Check sheet for the modelled part. Datum: model origin and axes. Units: mm. Face numbers are marked on the shaded views. A direction names the side the tool comes from. Give positions to 0.01 mm unless a question says otherwise; leave off trailing zeros. Order: outer loops, then holes, each group sorted by start corner. A loop starts at its lowest first (then second) coordinate and runs counter-clockwise, first axis right, second up. Notation, with made-up numbers: M 12.25,23 L 65.25,23 A9 cw 65.25,38 Z; hole C 82.25,5 d4. An arc over 180 degrees is marked long. Return JSON: item names as keys, results as strings. Group by question number.
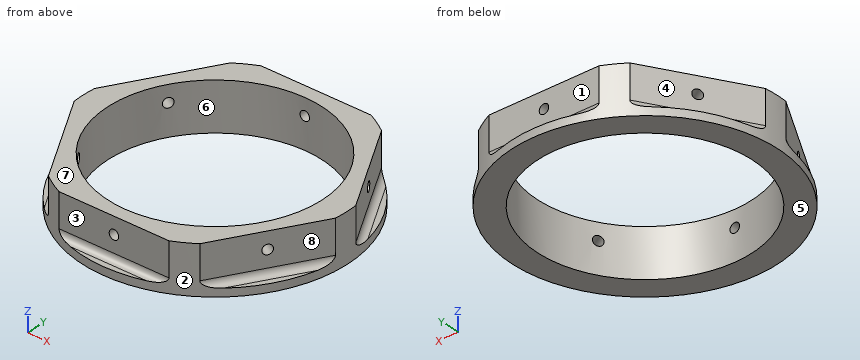
from build123d import *

# Parameters (mm, degrees)
SZKIC2_R                    = 46.017617149
DODANIE_WYCI_GNI_CIE1_DEPTH = 2.5
DODANIE_WYCI_GNI_CIE2_DEPTH = 15
SZKIC3_R                    = 46.5
SZKIC3_R_2                  = 42.5
WYTNIJ_WYCI_GNI_CIE3_DEPTH  = 10
SZKIC8_R                    = 33.35
WYTNIJ_WYCI_GNI_CIE2_DEPTH  = 62.947558467
ZAOKR_GLENIE2_R             = 2
SZKIC9_R                    = 1.5
WYTNIJ_WYCI_GNI_CIE4_DEPTH  = 10
SZYK_KO_OWY1_COUNT          = 6
SZKIC10_R                   = 50
SZKIC10_R_2                 = 41.3
WYTNIJ_WYCI_GNI_CIE5_DEPTH  = 62.947558491


with BuildPart() as part:
    # Szkic2 → Dodanie-wyci_gni_cie1 (new body)
    with BuildSketch(Plane.XY):
        Circle(SZKIC2_R)
    extrude(amount=DODANIE_WYCI_GNI_CIE1_DEPTH)

    # Szkic2_3 → Dodanie-wyci_gni_cie2 (add)
    with BuildSketch(Plane.XY):
        with BuildLine():
            ThreePointArc((17.776388835, -37.5), (20.75, -35.940054257), (23.587758225, -34.144804318))
            Line((23.587758225, -34.144804318), (41.364147059, -3.355195682))
            ThreePointArc((41.364147059, -3.355195682), (41.466022856, -1.67897246), (41.5, 0))
            ThreePointArc((41.5, 0), (41.466022856, 1.67897246), (41.364147059, 3.355195682))
            Line((41.364147059, 3.355195682), (23.587758225, 34.144804318))
            ThreePointArc((23.587758225, 34.144804318), (20.75, 35.940054257), (17.776388835, 37.5))
            Line((17.776388835, 37.5), (-17.776388835, 37.5))
            ThreePointArc((-17.776388835, 37.5), (-20.75, 35.940054257), (-23.587758225, 34.144804318))
            Line((-23.587758225, 34.144804318), (-41.364147059, 3.355195682))
            ThreePointArc((-41.364147059, 3.355195682), (-41.5, 0), (-41.364147059, -3.355195682))
            Line((-41.364147059, -3.355195682), (-23.587758225, -34.144804318))
            ThreePointArc((-23.587758225, -34.144804318), (-20.75, -35.940054257), (-17.776388835, -37.5))
            Line((-17.776388835, -37.5), (17.776388835, -37.5))
        make_face()
    extrude(amount=DODANIE_WYCI_GNI_CIE2_DEPTH)

    # Szkic3 → Wytnij-wyci_gni_cie3 (cut)
    with BuildSketch(Plane(origin=(0, 0, 2.5), x_dir=(-1, 0, 0), z_dir=(0, 0, -1))):
        Circle(SZKIC3_R)
        with Locations(Location((0, 0, 0), (0, 0, 180))):
            Circle(SZKIC3_R_2, mode=Mode.SUBTRACT)
    extrude(amount=WYTNIJ_WYCI_GNI_CIE3_DEPTH, mode=Mode.SUBTRACT)

    # Szkic8 → Wytnij-wyci_gni_cie2 (cut, through all)
    with BuildSketch(Plane.XY.offset(15)):
        Circle(SZKIC8_R)
    extrude(amount=-WYTNIJ_WYCI_GNI_CIE2_DEPTH, mode=Mode.SUBTRACT)

    # Zaokr_glenie2
    zaokr_glenie2_edges = [part.edges().sort_by_distance(p)[0] for p in [
        (32.475952642, -18.75, 2.5),
        (0, -37.5, 2.5),
        (-32.475952642, -18.75, 2.5),
        (-32.475952642, 18.75, 2.5),
        (0, 37.5, 2.5),
        (32.475952642, 18.75, 2.5),
    ]]
    fillet(zaokr_glenie2_edges, radius=ZAOKR_GLENIE2_R)

    # Szkic9 → Wytnij-wyci_gni_cie4 (cut)
    with BuildSketch(Plane(origin=(-32.475952642, -18.75, 0), x_dir=(0, 0, 1), z_dir=(-0.8660254037844386, -0.5000000000000001, 0))):
        with Locations(Location((9.75, 0, 0), (0, 0, 270))):
            Circle(SZKIC9_R)
    wytnij_wyci_gni_cie4 = extrude(amount=-WYTNIJ_WYCI_GNI_CIE4_DEPTH, mode=Mode.SUBTRACT)

    # Szyk ko_owy1: Wytnij-wyci_gni_cie4 ×6 about axis
    szyk_ko_owy1_axis = Axis((0, 0, 15), (0, 0, -1))
    for i in range(1, SZYK_KO_OWY1_COUNT):
        add(wytnij_wyci_gni_cie4.rotate(szyk_ko_owy1_axis, i * 360 / SZYK_KO_OWY1_COUNT), mode=Mode.SUBTRACT)

    # Szkic10 → Wytnij-wyci_gni_cie5 (cut, through all)
    with BuildSketch(Plane.XY.offset(15)):
        Circle(SZKIC10_R)
        Circle(SZKIC10_R_2, mode=Mode.SUBTRACT)
    extrude(amount=-WYTNIJ_WYCI_GNI_CIE5_DEPTH, mode=Mode.SUBTRACT)


solid = part.part
1) Sectioned sample at B-B on y = 0. Record the boundary of the cut face in (x, z).
2) Tool access check on the marked faces 1, 2, 3, 4 and 5. Record the directions out of +Z, -Z, +X, -X, +Y, -Y that give a thin tool (end or side, any length) a straight path to the whole face; none if there is none.
3) Sectioned sample at C-C on z = 6. Record the boundary of the cut face in (x, y).
4) Release check for a two-part mould opening along X. For the marked faces 6, 7 and 8 record: released by +X, released by -X, zero draft, split by the parting line, or undercut.
5) Depth check by flat-ended pin: P1, Ø0.9, axis at x = 4, y = 40, coming from the +Z side; P2, Ø3, axis at x = -1.5, z = 9, coming from the +Y side; P3, Ø3, axis at x = -7.5, z = 11, coming from the -Y side. Enter the tip coordinate at first touch or a pass-through.
6) Material ranges on line 1 along Y through (x, z) = (1, 5.5) (3 decimals); line 2 along Y through (x, z) = (1, 2) (3 decimals); line 3 along Z through (x, y) = (0, -34), recorded low to high.
7) Sectioned sample at D-D on x = -18.5. Record the boundary of the cut face in (y, z), then the cut area to 3 significant figures.
8) Sectioned sample at A-A on x = 0. Record the boundary of the cut face in (y, z).
Reply:
{
 "1": {"outline": "M -41.3,0 L -33.35,0 L -33.35,15 L -41.3,15 Z; M 33.35,0 L 41.3,0 L 41.3,15 L 33.35,15 Z"},
 "2": {"face 1": "+Z, +X, -X, +Y", "face 2": "+Z, -Z", "face 3": "+Z, +X, -X, -Y", "face 4": "+Z, -X, +Y", "face 5": "-Z, +X, -X, +Y, -Y"},
 "3": {"outline": "M -41.13,-3.76 L -23.82,-33.74 A41.3 ccw -17.3,-37.5 L 17.3,-37.5 A41.3 ccw 23.82,-33.74 L 41.13,-3.76 A41.3 ccw 41.13,3.76 L 23.82,33.74 A41.3 ccw 17.3,37.5 L -17.3,37.5 A41.3 ccw -23.82,33.74 L -41.13,3.76 A41.3 ccw Z; hole C 0,0 d66.7"},
 "4": {"face 6": "undercut", "face 7": "zero draft", "face 8": "released by +X"},
 "5": {"P1": "z = 2.5", "P2": "y = 37.5", "P3": "y = -37.5"},
 "6": {"line 1": "-37.5 to -33.335, 33.335 to 37.5", "line 2": "-41.288 to -33.335, 33.335 to 41.288", "line 3": "0 to 8.25, 11.25 to 15"},
 "7": {"outline": "M -36.92,0 L -27.75,0 L -27.75,15 L -36.92,15 Z; M 27.75,0 L 36.92,0 L 36.92,15 L 27.75,15 Z", "area": "275 mm^2"},
 "8": {"outline": "M -41.3,0 L -33.35,0 L -33.35,8.25 L -37.5,8.25 L -37.5,4.5 A2 cw -39.5,2.5 L -41.3,2.5 Z; M -37.5,11.25 L -33.35,11.25 L -33.35,15 L -37.5,15 Z; M 33.35,0 L 41.3,0 L 41.3,2.5 L 39.5,2.5 A2 cw 37.5,4.5 L 37.5,8.25 L 33.35,8.25 Z; M 33.35,11.25 L 37.5,11.25 L 37.5,15 L 33.35,15 Z"}
}
